from build123d import *

# Parameters (mm, degrees)
F1_DEPTH = 50
F2_R     = 3
F3_DEPTH = 25


with BuildPart() as f1:
    # F0 (on Front) → F1 (new body)
    with BuildSketch(Plane.XZ):
        Polygon((-17.5, 12.5), (-17.5, -12.5), (-12.5, -12.5), (-12.5, 2.5), (12.5, 2.5), (12.5, -12.5), (17.5, -12.5), (17.5, 12.5), align=None)
    extrude(amount=F1_DEPTH)

    # F2 (on face) → F3 (cut)
    with BuildSketch(Plane.XY.offset(12.5)):
        with Locations((0, -10)):
            Circle(F2_R)
        with Locations((0, -40)):
            Circle(F2_R)
    extrude(amount=-F3_DEPTH, mode=Mode.SUBTRACT)


solid = f1.part
Part model, mm, in its own coordinate system. A direction names the side the tool comes from. Give positions to 0.01 mm unless a question says otherwise; leave off trailing zeros. Loops run counter-clockwise (first coordinate to the right, second up) from the corner with the lowest first, then second, coordinate; pieces in that order, holes last. Notation, with made-up numbers: (54, -16) -> (92, -16) arc R30 ccw to (92, 18) -> close; hole circle Ø2 at (27.25, -35.75). An arc over 180 degrees is marked (long way). Write each question's results on one line, items separated by ' | '. Start each with the question number.
Q1. Pull direction X, two halves, no side cores. Call faces 1 (the face through (17.5, -25, 0)), 2 (the face through (12.5, -25, -5)), 3 (the face through (-17.5, -25, 0)): +X half, -X half, draft (parallel to the pull), parting line (faces both ways), or undercut.
Q2. Wall check: L1, parallel to Y at x = 0, z = 4.75; L2, parallel to X at y = -11.5, z = -5; L3, parallel to Z at x = 6, y = -31. Give the ranges that are in metal, low to high.
Q3. Pin check, flat tip, straight feed: P1, Ø1, axis at x = 8, y = -14.5, coming from the -Z side. Stop position of the tip, or through.
Q4. Band-saw the part on B-B on z = -11. List the corners of the cut face in (x, y), plus the area to 3 significant figures.
Q5. Band-saw the part on C-C on y = -10. List the corners of the cut face in (x, z), plus the area to 3 significant figures.
Q6. Which spindle directions (+Z, -Z, +X, -X, +Y, -Y) get a long thin tool onto all of the face, cutting with end or side? Do faces 4 (the face through (-15, -25, -12.5)), 5 (the face through (-12.5, -25, -5)). Say none if no direction does.
Q7. Band-saw the part on D-D on z = 4.5. List the corners of the cut face in (x, y).
Q8. Band-saw the part on A-A on x = 0. List the corners of the cut face in (y, z).
Results are:
1) face 1: +X half | face 2: undercut | face 3: -X half
2) L1: y = -50 to -43, -37 to -13, -7 to 0 | L2: x = -17.5 to -12.5, 12.5 to 17.5 | L3: z = 2.5 to 12.5
3) P1: stops at z = 2.5
4) outline: (-17.5, -50) -> (-12.5, -50) -> (-12.5, 0) -> (-17.5, 0) -> close; (12.5, -50) -> (17.5, -50) -> (17.5, 0) -> (12.5, 0) -> close | area: 500 mm²
5) outline: (-17.5, -12.5) -> (-12.5, -12.5) -> (-12.5, 2.5) -> (-3, 2.5) -> (-3, 12.5) -> (-17.5, 12.5) -> close; (3, 2.5) -> (12.5, 2.5) -> (12.5, -12.5) -> (17.5, -12.5) -> (17.5, 12.5) -> (3, 12.5) -> close | area: 440 mm²
6) face 4: -Z, +X, -X, +Y, -Y | face 5: -Z, +Y, -Y
7) outline: (-17.5, -50) -> (17.5, -50) -> (17.5, 0) -> (-17.5, 0) -> close; hole circle Ø6 at (0, -40); hole circle Ø6 at (0, -10)
8) outline: (-50, 2.5) -> (-43, 2.5) -> (-43, 12.5) -> (-50, 12.5) -> close; (-37, 2.5) -> (-13, 2.5) -> (-13, 12.5) -> (-37, 12.5) -> close; (-7, 2.5) -> (0, 2.5) -> (0, 12.5) -> (-7, 12.5) -> close
